```python
from build123d import *

# Parameters (mm, degrees)
BOSS_EXTRUDE2_START     = 12.827
BOSS_EXTRUDE2_DEPTH     = 6.35
F_1_4_CLEARANCE_HOLE2_D = 7.14248
FILLET2_R               = 6.35


with BuildPart() as part:
    # Sketch5 → Boss-Extrude2 (new body)
    with BuildSketch(Plane(origin=(0, 144.904574554, 0), x_dir=(-1, 0, 0), z_dir=(0, -1, 0)).offset(BOSS_EXTRUDE2_START)):
        with BuildLine():
            Line((-124.491812484, -1137.975334154), (-124.491812484, -1087.175334154))
            ThreePointArc((-124.491812484, -1087.175334154), (-114.966812484, -1077.650334154), (-105.441812484, -1087.175334154))
            Line((-105.441812484, -1087.175334154), (-105.441812484, -1103.050334154))
            Line((-105.441812484, -1103.050334154), (-64.166812484, -1103.050334154))
            ThreePointArc((-64.166812484, -1103.050334154), (-54.641812484, -1112.575334154), (-64.166812484, -1122.100334154))
            Line((-64.166812484, -1122.100334154), (-70.516812484, -1122.100334154))
            Line((-70.516812484, -1122.100334154), (-70.516812484, -1163.375334154))
            ThreePointArc((-70.516812484, -1163.375334154), (-80.041812484, -1172.900334154), (-89.566812484, -1163.375334154))
            Line((-89.566812484, -1163.375334154), (-89.566812484, -1122.100334154))
            Line((-89.566812484, -1122.100334154), (-105.441812484, -1122.100334154))
            Line((-105.441812484, -1122.100334154), (-105.441812484, -1137.975334154))
            ThreePointArc((-105.441812484, -1137.975334154), (-114.966812484, -1147.500334154), (-124.491812484, -1137.975334154))
        make_face()
    extrude(amount=BOSS_EXTRUDE2_DEPTH)

    # 1/4 Clearance Hole2 (through all)
    with Locations(Plane(origin=(0, 125.727574554, 0), x_dir=(-1, 0, 0), z_dir=(0, -1, 0))):
        with Locations((-114.966812484, -1087.175334154), (-114.966812484, -1137.975334154), (-114.966812484, -1112.575334154), (-89.566812484, -1112.575334154), (-64.166812484, -1112.575334154), (-80.041812484, -1137.975334154), (-80.041812484, -1163.375334154)):
            Hole(F_1_4_CLEARANCE_HOLE2_D / 2)

    # Fillet2
    fillet2_edges = [part.edges().sort_by_distance(p)[0] for p in [
        (105.441812484, 128.902574554, 1103.050334154),
        (70.516812484, 128.902574554, 1122.100334154),
        (89.566812484, 128.902574554, 1122.100334154),
        (105.441812484, 128.902574554, 1122.100334154),
    ]]
    fillet(fillet2_edges, radius=FILLET2_R - 0.0001)  # a hair under: the kernel refuses the full size


solid = part.part
```
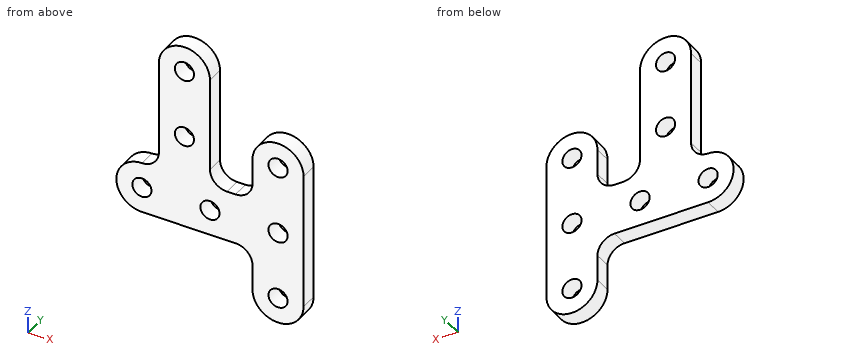
The model under review builds one solid part; all positions refer to its coordinate system, in mm. Round coordinates to 2 decimals unless told otherwise and drop trailing zeros. Order: outer loops, then holes, each group sorted by start corner. A loop starts at its lowest first (then second) coordinate and runs counter-clockwise, first axis right, second up.
(1) Take a section at C-C, the plane y = 129.5. Count the separate pieces of the cut face and the enclosed holes in it, plus the area to 3 significant figures.
Working result:
separate pieces: 1
enclosed holes: 7
area: 2,860 mm2
(2) Take a section at A-A, the plane z = 1130.5. State the section outline as (x, y) points.
Working result:
outline: (70.52, 125.73) - (89.57, 125.73) - (89.57, 132.08) - (70.52, 132.08) - close; (105.44, 125.73) - (124.49, 125.73) - (124.49, 132.08) - (105.44, 132.08) - close
(3) Wall thickness on L1, parallel to X at y = 127.5, z = 1138; L2, parallel to X at y = 129.5, z = 1132.5; L3, parallel to X at y = 129, z = 1140: over which ranges is each line inside the solid? List them lowest first.
Working result:
L1: x = 70.52 to 76.47, 83.61 to 89.57, 105.44 to 111.4, 118.54 to 124.49
L2: x = 70.52 to 89.57, 105.44 to 124.49
L3: x = 70.52 to 77.1, 82.98 to 89.57, 105.66 to 112.02, 117.91 to 124.27
(4) Take a section at D-D, the plane x = 117.5. State the section outline as (y, z) points.
Working result:
outline: (125.73, 1077.99) - (132.08, 1077.99) - (132.08, 1084.66) - (125.73, 1084.66) - close; (125.73, 1089.69) - (132.08, 1089.69) - (132.08, 1110.06) - (125.73, 1110.06) - close; (125.73, 1115.09) - (132.08, 1115.09) - (132.08, 1135.46) - (125.73, 1135.46) - close; (125.73, 1140.49) - (132.08, 1140.49) - (132.08, 1147.16) - (125.73, 1147.16) - close
(5) Take a section at B-B, the plane x = 62.5. State the section outline as (y, z) points.
Working result:
outline: (125.73, 1103.2) - (132.08, 1103.2) - (132.08, 1109.42) - (125.73, 1109.42) - close; (125.73, 1115.73) - (132.08, 1115.73) - (132.08, 1121.95) - (125.73, 1121.95) - close
(6) For P1, Ø3, axis at y = 129.5, z = 1131, coming from the -X side; P2, Ø1.5, axis at x = 117.5, y = 128.5, coming from the +Z side; P3, Ø3, axis at y = 130, z = 1140, coming from the +X side, all flat-tipped, find the tip position at first contact; note any pin that passes through.
Working result:
P1: stops at x = 70.52
P2: stops at z = 1147.33
P3: stops at x = 124.48
